Autodesk Inventor part; units mm, degrees
ref_plane "Work Plane1" through (8, 6, 40) normal (0, -1, 0) x (1, 0, 0)
ref_plane "YZ Plane" through (0, 0, 0) normal (1, 0, 0) x (0, 1, 0)
ref_plane "XZ Plane" through (0, 0, 0) normal (0, 1, 0) x (-1, 0, 0)
sketch "Sketch1" plane through (0, 0, 0) normal (1, 0, 0) x (0, 1, 0)
  arc A0 (26.4575, -30) -> (0, 40) centre (0, 0) ccw
  line L0 (0, 40) -> (0, -30)
  line L1 (0, -30) -> (26.4575, -30)
  arc A1 (0, 40) -> (26.4575, -30) centre (0, 0) ccw construction
  dimension "d0" = 80
  dimension "d1" = 70
extrude "Extrusion1" add sketch "Sketch1" along normal blind 62
fillet "Fillet1" radius 8 2 edges at (0, 37.4166, 14.1421) (62, 37.4166, 14.1421)
sketch "Sketch2" plane through (0, 0, -30) normal (0, -1, 0) x (1, 0, 0)
  circle A0 centre (31, -23.9392) radius 9.6
  line L0 (0, 0) -> (62, 0)
  line L1 (31, -23.9392) -> (31, 0) construction
  line L2 (34.5, 0) -> (27.5, 0)
  line L3 (27.5, 0) -> (27.5, -15)
  line L4 (34.5, 0) -> (34.5, -15)
  point P0 (0, 30)
  dimension "d6" = 19.2
  dimension "d7" = 3.5
  dimension "d8" = 3.5
  dimension "d61" = 15
extrude "Extrusion2" add sketch "Sketch2" against normal blind 25
sketch "Sketch3" plane through (34.5, 0, -30) normal (1, 0, 0) x (0, 0, -1)
  line L0 (0, 25) -> (15, 25)
  line L1 (0, 11.1355) -> (0, 26.4575)
  arc A0 (1.225, 25) -> (0, 26.4575) centre (-30.0052, -0.0046) ccw
  arc A1 (0, 26.4575) -> (-70, 0) centre (-30, 0) ccw
  line L2 (0, 26.4575) -> (1.225, 25) construction
  point P0 (-30, 0)
  dimension "d13" = 1.225
extrude "Extrusion3" add sketch "Sketch3" against normal up to surface (7 mm away)
sketch "Sketch4" plane through (0, 0, -30) normal (0, -1, 0) x (1, 0, 0)
  line L0 (58.9, 60.95) -> (51.4, 60.95)
  line L1 (18.3, 60.95) -> (18.3, 19.35)
  line L2 (58.9, 19.35) -> (58.9, 60.95)
  line L3 (58.9, 37.4) -> (60.4, 37.4)
  line L4 (60.4, 37.4) -> (60.4, 30)
  line L5 (60.4, 22.6) -> (58.9, 22.6)
  line L6 (58.9, 22.6) -> (58.9, 37.4)
  line L7 (60.4, 35) -> (62, 35)
  line L8 (62, 35) -> (62, 30)
  line L9 (62, 25) -> (60.4, 25)
  line L10 (60.4, 25) -> (60.4, 35)
  line L11 (47.7, 19.35) -> (47.7, 12.25)
  line L12 (47.7, 12.25) -> (51.4, 12.25)
  line L13 (51.4, 12.25) -> (51.4, 19.35)
  line L14 (22.2, 19.35) -> (22.2, 13.35)
  line L15 (22.2, 13.35) -> (27.6, 13.35)
  line L16 (27.6, 13.35) -> (27.6, 19.35)
  line L17 (47.7, 60.95) -> (47.7, 68.05)
  line L18 (47.7, 68.05) -> (51.4, 68.05)
  line L19 (51.4, 68.05) -> (51.4, 60.95)
  line L20 (47.7, 60.95) -> (18.3, 60.95)
  line L21 (51.4, 19.35) -> (58.9, 19.35)
  line L22 (18.3, 19.35) -> (22.2, 19.35)
  line L23 (27.6, 19.35) -> (47.7, 19.35)
  line L24 (62, 62) -> (62, 0)
  line L25 (54, 0) -> (54, 70)
  line L26 (0, 30) -> (48.0104, 30) construction
  line L27 (62, 30) -> (58.9, 30)
  line L28 (62, 30) -> (62, 25)
  line L29 (60.4, 30) -> (60.4, 22.6)
  dimension "d16" = 40.6
  dimension "d17" = 41.6
  dimension "d18" = 10
  dimension "d19" = 14.8
  dimension "d20" = 1.6
  dimension "d21" = 1.5
  dimension "d22" = 10.65
  dimension "d23" = 3.7
  dimension "d24" = 7.5
  dimension "d25" = 7.1
  dimension "d26" = 7.1
  dimension "d27" = 3.9
  dimension "d28" = 5.4
  dimension "d29" = 6
  dimension "d30" = 5
extrude "Extrusion4" cut sketch "Sketch4" against normal blind 10.6 contours L2 L21 L25 L0 | L25 L21 L13 L12 L11 L23 L16 L15 L14 L22 L1 L20 L17 L18 L19 L0
revolve "Revolution1" cut sketch "Sketch4" angle 360 about axis through (62, 0, 0) along (-1, 0, 0) contours L27 L10 L29 L5 L2 | L27 L24 L9 L10
sketch "Sketch5" plane through (0, 0, -30) normal (0, -1, 0) x (1, 0, 0)
  line L0 (0, 30) -> (14.3, 30)
  line L1 (14.3, 30) -> (14.3, 17.6)
  line L2 (14.3, 17.6) -> (0, 17.6)
  line L3 (0, 17.6) -> (0, 30)
  dimension "d34" = 24.8
  dimension "d35" = 14.3
revolve "Revolution2" cut sketch "Sketch5" angle 360 about axis through (0, 0, 0) along (1, 0, 0)
sketch "Sketch6" plane through (8, 0, 40) normal (0, -1, 0) x (1, 0, 0)
  line L0 (6.3, -52.4) -> (-8, -52.4)
  line L1 (6.3, -27.6) -> (6.3, -52.4)
  line L2 (-8, -27.6) -> (6.3, -27.6)
  line L3 (-8, -52.4) -> (-8, -27.6)
  line L4 (6.3, -52.4) -> (-3, -52.4)
  line L5 (-3, -52.4) -> (-3, -65.75)
  line L6 (-3, -65.75) -> (6.3, -65.75)
  line L7 (6.3, -65.75) -> (6.3, -52.4)
  line L8 (-8, -70) -> (19.5, -70)
  line L9 (-3, -52.4) -> (6.3, -52.4)
  line L10 (6.3, -52.4) -> (6.3, -40)
  line L11 (6.3, -40) -> (-3, -40)
  line L12 (-3, -40) -> (-3, -52.4)
  point P0 (-8, -40)
  dimension "d38" = 5
  dimension "d39" = 4.25
extrude "Extrusion5" cut sketch "Sketch6" against normal blind 12.4 contours L7 L6 L5 L0 | L0 L12 L11 L1
sketch "Sketch7" plane through (8, 0, 40) normal (0, -1, 0) x (1, 0, 0)
  line L0 (-3, -65.75) -> (-3, -52.4)
  line L1 (-3, -52.4) -> (-8, -52.4)
  line L2 (-8, -52.4) -> (-8, -70)
  line L3 (-8, -70) -> (19.5, -70)
  line L4 (19.5, -70) -> (19.5, -85)
  arc A0 (19.5, -85) -> (26.5, -85) centre (23, -93.9392) ccw
  line L5 (26.5, -85) -> (26.5, -70)
  line L6 (26.5, -70) -> (54, -70)
  line L7 (54, -45) -> (54, -70)
  line L8 (54, -45) -> (52.4, -45)
  line L9 (52.4, -45) -> (52.4, -47.4)
  line L10 (52.4, -47.4) -> (50.9, -47.4)
  line L11 (50.9, -47.4) -> (50.9, -50.65)
  line L12 (50.9, -50.65) -> (43.4, -50.65)
  line L13 (43.4, -50.65) -> (43.4, -57.75)
  line L14 (43.4, -57.75) -> (39.7, -57.75)
  line L15 (39.7, -57.75) -> (39.7, -50.65)
  line L16 (39.7, -50.65) -> (19.6, -50.65)
  line L17 (19.6, -50.65) -> (19.6, -56.65)
  line L18 (19.6, -56.65) -> (14.2, -56.65)
  line L19 (14.2, -56.65) -> (14.2, -50.65)
  line L20 (14.2, -50.65) -> (10.3, -50.65)
  line L21 (10.3, -50.65) -> (10.3, -9.05)
  line L22 (10.3, -9.05) -> (39.7, -9.05)
  line L23 (39.7, -9.05) -> (39.7, -1.95)
  line L24 (39.7, -1.95) -> (43.4, -1.95)
  line L25 (43.4, -1.95) -> (43.4, -9.05)
  line L26 (43.4, -9.05) -> (50.9, -9.05)
  line L27 (50.9, -9.05) -> (50.9, -32.6)
  line L28 (50.9, -32.6) -> (52.4, -32.6)
  line L29 (52.4, -32.6) -> (52.4, -35)
  line L30 (52.4, -35) -> (54, -35)
  line L31 (54, -8) -> (54, -35)
  arc A1 (54, -8) -> (46, 0) centre (46, -8) ccw
  line L32 (0, 0) -> (46, 0)
  arc A2 (0, 0) -> (-8, -8) centre (0, -8) ccw
  line L33 (-8, -8) -> (-8, -27.6)
  line L34 (-8, -27.6) -> (6.3, -27.6)
  line L35 (6.3, -27.6) -> (6.3, -65.75)
  line L36 (6.3, -65.75) -> (-3, -65.75)
  circle A3 centre (1.15, -9.15) radius 2
  circle A4 centre (34, -60.325) radius 2
  circle A5 centre (48, -60.325) radius 2
  point P0 (-8, -40)
  dimension "d42" = 4
  dimension "d43" = 4
  dimension "d44" = 18.3
  dimension "d45" = 9.15
  dimension "d46" = 9.15
  dimension "d47" = 19.35
  dimension "d48" = 9.675
  dimension "d49" = 20
  dimension "d52" = 4
  dimension "d53" = 6
  dimension "d54" = 9.675
extrude "Extrusion6" cut sketch "Sketch7" against normal through all contours A3 | A4 | A5
ref_plane "Work Plane1" through (8, 6, 40) normal (0, -1, 0) x (1, 0, 0)
sketch "Sketch8" plane through (8, 6, 40) normal (0, -1, 0) x (1, 0, 0)
  circle A0 centre (48, -60.325) radius 2
  circle A1 centre (34, -60.325) radius 2
  circle A2 centre (1.15, -9.15) radius 2
  circle A3 centre (1.15, -9.15) radius 3.75
  circle A4 centre (34, -60.325) radius 3.75
  circle A5 centre (48, -60.325) radius 3.75
  point P0 (-8, -40)
  dimension "d56" = 7.5
  dimension "d57" = 7.5
  dimension "d58" = 7.5
extrude "Extrusion7" cut sketch "Sketch8" against normal through all contours A0 | A1 | A2 | A3 | A4 | A5
sketch "Sketch9" plane through (34.5, 0, -30) normal (1, 0, 0) x (0, 0, -1)
  circle A0 centre (9.225, 12.5) radius 2
  line L0 (1.225, 25) -> (15, 25)
  line L1 (15, 0) -> (15, 25)
  line L2 (0, 0) -> (0, 11.1355)
  point P0 (-30, 0)
  point P1 (8.1125, 25)
  dimension "d62" = 4
  dimension "d63" = 12.5
  dimension "d67" = 9.225
extrude "Extrusion8" cut sketch "Sketch9" against normal through all
chamfer "Chamfer1" distance 10 angle 45 1 edges at (24.9, 0, -16.65)
equation "\"d26\" = d25"
equation "\"d45\" = 0.5 * d44"
equation "\"d46\" = d45"
equation "\"d48\" = 0.5 * d47"
equation "\"d54\" = d48"
properties part number "Arm_1Up"
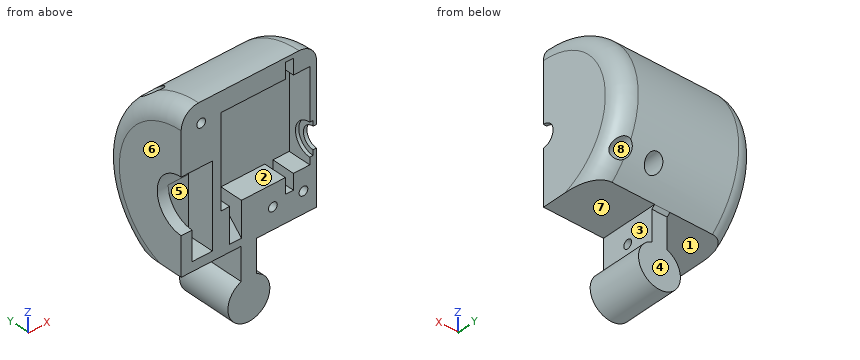
Verification items for the finished model (mm, model axes). Face numbers are marked on the shaded views. A direction names the side the tool comes from. Coordinates: 2 decimals unless noted, no trailing zeros. Write each loop counter-clockwise with the first axis right and the second up, starting at its lowest first coordinate (ties: lowest second). Pieces come first, ordered by that corner, then holes. Notation, with made-up numbers: M 15,-11.75 L 28,-11.75 A30 cw 28,25.25 Z; hole C 57,42 d10. An arc over 180 degrees is marked long. Use a Markdown table: item, result.
Q1. Draft check along X on the marked faces 5, 6, 7 and 8. Enter one of: +X half, -X half, draft (parallel to the pull), parting line (faces both ways), or undercut.
Reply:
| item | result |
|---|---|
| face 5 | undercut |
| face 6 | -X half |
| face 7 | draft |
| face 8 | undercut |
Q2. Thickness scan on line 1 (Z direction, x = 42, y = 24) (3 decimals); line 2 (Z direction, x = 55, y = 2.5); line 3 (Z direction, x = 42, y = 4.1) (3 decimals). Record the ranges inside material, lowest first.
Reply:
| item | result |
|---|---|
| line 1 | z = -30 to -24.075, -16.575 to 32 |
| line 2 | z = -30 to -22.06, -18.59 to -10.65, 30.95 to 39.86 |
| line 3 | z = -30 to -22.325, -18.325 to -10.65, 30.95 to 39.789 |
Q3. Go/stop test with flat-tipped pins: P1, Ø1.8, axis at x = 49.5, y = 4, coming from the -Z side; P2, Ø6, axis at x = 42, z = -20.325, coming from the +Y side; P3, Ø21, axis at x = 17, y = 10, coming from the -Z side. Record where each tip stops, or that it passes through.
Reply:
| item | result |
|---|---|
| P1 | stops at z = -30 |
| P2 | stops at y = 6 |
| P3 | stops at z = -62.88 |
Q4. Sectioned sample at D-D, the plane z = -35.5. Record the boundary of the cut face in (x, y), plus the area to 3 significant figures.
Reply:
| item | result |
|---|---|
| outline | M 27.5,0 L 34.5,0 L 34.5,25 L 27.5,25 Z |
| area | 175 mm² |
Q5. Set-up check for the marked faces 1, 2, 3 and 4: record each of +Z, -Z, +X, -X, +Y, -Y from which the full face is reachable in a straight line by a thin tool's end or side.
Reply:
| item | result |
|---|---|
| face 1 | -X, +Y, -Y |
| face 2 | -Y |
| face 3 | +X, +Y, -Y |
| face 4 | -Z, +X, -X, +Y |
Q6. Sectioned sample at C-C, the plane y = 8.5. Count the separate pieces of the cut face and the enclosed holes in it, plus the area to 3 significant figures.
Reply:
| item | result |
|---|---|
| separate pieces | 1 |
| enclosed holes | 4 |
| area | 2,320 mm² |
